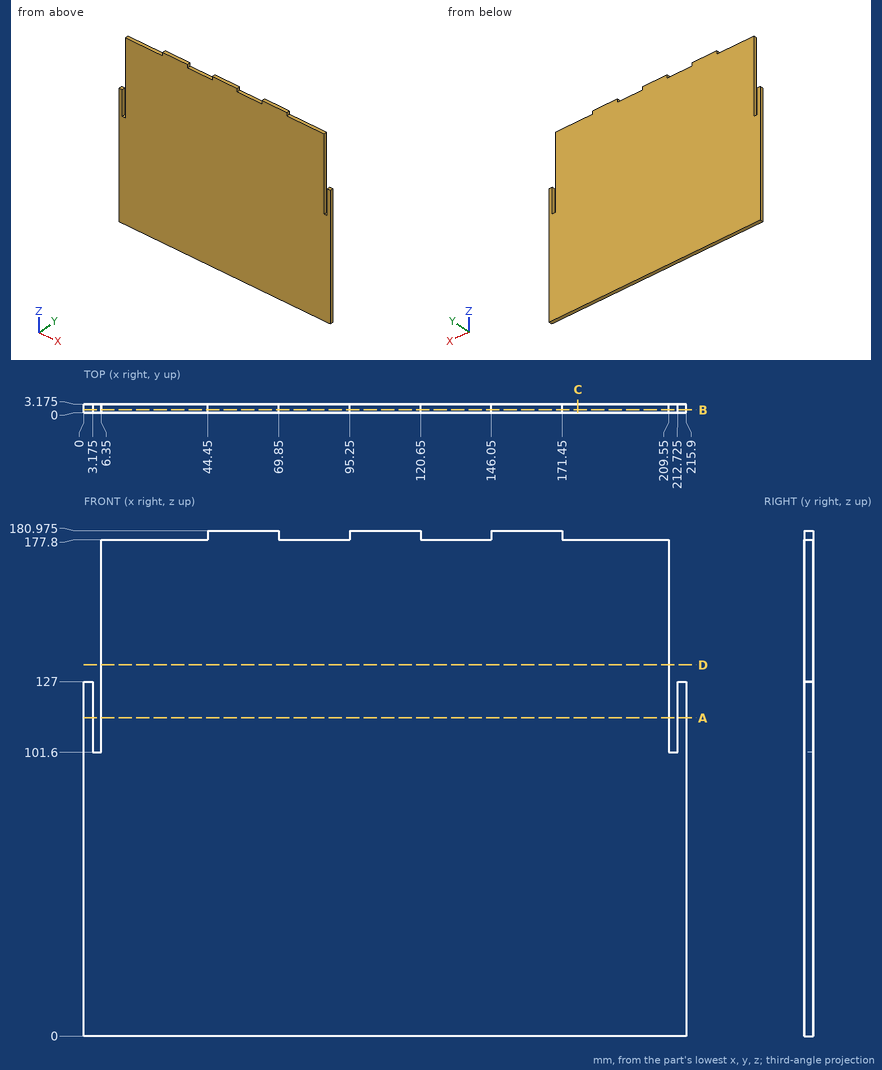
Design review of the part shown in the three views and the two pictorial views. Dimensions are in mm from the part's minimum x, y and z. Round coordinates to 2 decimals unless told otherwise and drop trailing zeros. Write each loop counter-clockwise with the first axis right and the second up, starting at its lowest first coordinate (ties: lowest second). Pieces come first, ordered by that corner, then holes. Notation, with made-up numbers: (3.25, 74) - (58.25, 74) arc R21 ccw to (58.25, 108) - close; hole circle Ø8 at (68.5, -1). An arc over 180 degrees is marked (long way). Answer as CSV lines item,"result". Start each with the question number.
(1) For pin 1 (1.5 mm diameter, centred on y = 2, z = 155.5, fed in from -X); pin 2 (1 mm diameter, centred on y = 2.5, z = 180, fed in from -X); pin 3 (1 mm diameter, centred on x = 136, y = 2, fed in from +Z), all flat-tipped, find the tip position at first contact; note any pin that passes through.
(2) Add section D-D, the plane z = 133. State the section outline as (x, y) points (3 decimals), plus the area to 3 significant figures.
(3) Add section B-B, the plane y = 1.1. State the section outline as (x, z) points (3 decimals), plus the area to 3 significant figures.
(4) Add section C-C, the plane x = 177. State the section outline as (y, z) points (3 decimals), plus the area to 3 significant figures.
(5) Add section A-A, the plane z = 114. State the section outline as (x, y) points (3 decimals), plus the area to 3 significant figures.
(6) For line 1 (X direction, y = 2.3, z = 111) (3 decimals); line 2 (Z direction, x = 135, y = 0.85); line 3 (X direction, y = 1.8, z = 139), list the stretches that pass through material, from the lowest coordinate up.
From the geometry:
1,pin 1,"stops at x = 6.35"
1,pin 2,"stops at x = 44.45"
1,pin 3,"stops at z = 177.8"
2,outline,"(6.35, 0) - (209.55, 0) - (209.55, 3.175) - (6.35, 3.175) - close"
2,area,"645 mm²"
3,outline,"(0, 0) - (215.9, 0) - (215.9, 127) - (212.725, 127) - (212.725, 101.6) - (209.55, 101.6) - (209.55, 177.8) - (171.45, 177.8) - (171.45, 180.975) - (146.05, 180.975) - (146.05, 177.8) - (120.65, 177.8) - (120.65, 180.975) - (95.25, 180.975) - (95.25, 177.8) - (69.85, 177.8) - (69.85, 180.975) - (44.45, 180.975) - (44.45, 177.8) - (6.35, 177.8) - (6.35, 101.6) - (3.175, 101.6) - (3.175, 127) - (0, 127) - close"
3,area,"37,800 mm²"
4,outline,"(0, 0) - (3.175, 0) - (3.175, 177.8) - (0, 177.8) - close"
4,area,"565 mm²"
5,outline,"(0, 0) - (3.175, 0) - (3.175, 3.175) - (0, 3.175) - close; (6.35, 0) - (209.55, 0) - (209.55, 3.175) - (6.35, 3.175) - close; (212.725, 0) - (215.9, 0) - (215.9, 3.175) - (212.725, 3.175) - close"
5,area,"665 mm²"
6,line 1,"x = 0 to 3.175, 6.35 to 209.55, 212.725 to 215.9"
6,line 2,"z = 0 to 177.8"
6,line 3,"x = 6.35 to 209.55"
